Part print with two shaded views. Sizes in mm from the minimum x, y, z corner. Round coordinates to 2 decimals unless told otherwise and drop trailing zeros. Order: outer loops, then holes, each group sorted by start corner. A loop starts at its lowest first (then second) coordinate and runs counter-clockwise, first axis right, second up. Notation, with made-up numbers: (-11.75, 12.5) -> (15.25, 12.5) arc R15 ccw to (15.25, 33.5) -> close; hole circle Ø3 at (58, 2). An arc over 180 degrees is marked (long way). Answer as a JSON object with one key per item and string values.
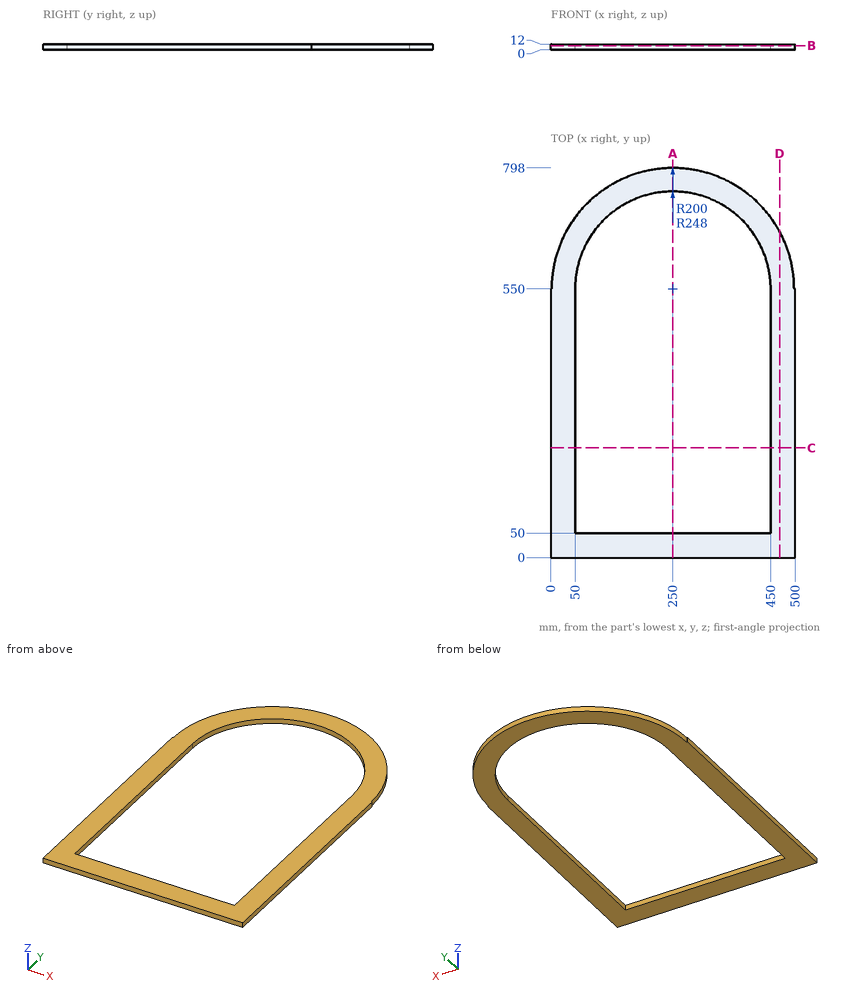
1) Cut at D-D, the plane x = 468.5. Give the cut face in (y, z), plus the area to 3 significant figures.
Checked values:
{"outline": "(0, 0) -> (667.31, 0) -> (667.31, 12) -> (0, 12) -> close", "area": "8,010 mm²"}
2) Cut at A-A, the plane x = 250. Give the cut face in (y, z).
Checked values:
{"outline": "(0, 0) -> (50, 0) -> (50, 12) -> (0, 12) -> close; (750, 0) -> (798, 0) -> (798, 12) -> (750, 12) -> close"}
3) Probe L1, parallel to X at y = 403, z = 10.5; L2, parallel to Y at x = 243.5, z = 5.5; L3, parallel to Y at x = 399.5, z = 2.5. List the from-to ranges inside material, lowest first. Write a range as from..to.
Checked values:
{"L1": "x = 0..50, 450..500", "L2": "y = 0..50, 749.89..797.91", "L3": "y = 0..50, 682.85..747.87"}
4) Cut at B-B, the plane z = 8.5. Give the cut face in (x, y), plus the area to 3 significant figures.
Checked values:
{"outline": "(0, 0) -> (500, 0) -> (500, 550) -> (498, 550) arc R248 ccw to (2, 550) -> (0, 550) -> close; hole (50, 50) -> (450, 50) -> (450, 550) arc R200 ccw to (50, 550) -> close", "area": "109,000 mm²"}
5) Flat gauge pin, fed straight in: pin 1 Ø1 at (x, z) = (0.5, 6.5) entering from +Y. Where does the tip first touch, or does it go through?
Checked values:
{"pin 1": "stops at y = 550"}
6) Cut at C-C, the plane y = 224.5. Give the cut face in (x, z).
Checked values:
{"outline": "(0, 0) -> (50, 0) -> (50, 12) -> (0, 12) -> close; (450, 0) -> (500, 0) -> (500, 12) -> (450, 12) -> close"}
